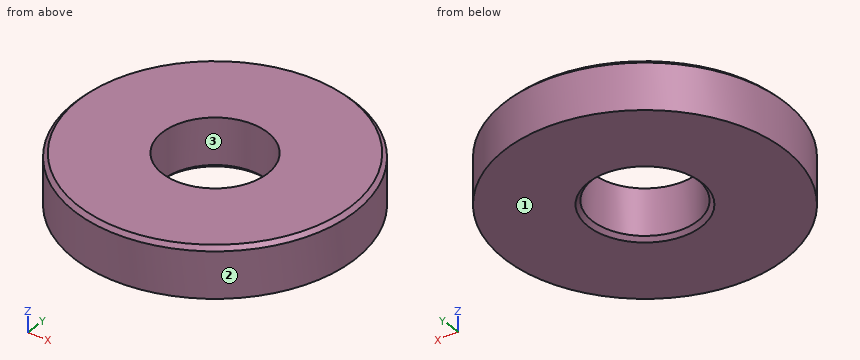
```python
from build123d import *

# Parameters (mm, degrees)
SKETCH_1_R      = 10.75
SKETCH_1_R_2    = 4.04
EXTRUDE_1_DEPTH = 3.85
CHAMFER_1_SIZE  = 0.3
CHAMFER_2_SIZE  = 0.3


with BuildPart() as part:
    # 草图1 → 凸台-拉伸1 (new body)
    with BuildSketch(Plane.XY):
        Circle(SKETCH_1_R)
        Circle(SKETCH_1_R_2, mode=Mode.SUBTRACT)
    extrude(amount=EXTRUDE_1_DEPTH)

    # 倒角1
    chamfer_1_edges = [part.edges().sort_by_distance(p)[0] for p in [
        (-10.75, 0, 3.85),
    ]]
    chamfer(chamfer_1_edges, length=CHAMFER_1_SIZE)

    # 倒角2
    chamfer_2_edges = [part.edges().sort_by_distance(p)[0] for p in [
        (-4.04, 0, 0),
    ]]
    chamfer(chamfer_2_edges, length=CHAMFER_2_SIZE)


solid = part.part
```
Source: CAD feature listing. Evaluate the final solid. Frame: model axes, mm. Face numbers are marked on the shaded views. Coordinates: 2 decimals unless noted, no trailing zeros. Loops run counter-clockwise (first coordinate to the right, second up) from the corner with the lowest first, then second, coordinate; pieces in that order, holes last. Notation, with made-up numbers: M 42.5,20 L 77.5,20 A15 ccw 77.5,34 Z; hole C 32.5,21.5 d2. An arc over 180 degrees is marked long. Put each result on its own line as item: value. Start each with the question number.
1) Cut plane C-C on z = 3.25. Return the cut outline in (x, y), then the cut area to 3 significant figures.
2) Ray query, L1, parallel to Y at x = 0, z = 3.05; L2, parallel to X at y = -0.25, z = 3.2; L3, parallel to X at y = 1, z = 3.5. Return the intervals inside material, ascending. Write a range as from..to.
3) Contact query for flat-ended pins moving along their axis: pin 1 Ø3 at (x, y) = (4, 3) entering from -Z; pin 2 Ø2 at (x, z) = (-3, 2) entering from +Y; pin 3 Ø1 at (x, z) = (2.5, 2) entering from -Y. Output: stop coordinate, or through.
4) Cut plane A-A on y = 0. Return the cut outline in (x, z), then the cut area to 3 significant figures.
5) Pull-direction query (X, two-part tool) for the marked faces 1, 2 and 3; classes: pulls with the +X half, pulls with the -X half, needs draft (parallel to the pull), parting line crosses it, or undercut.
The answers:
1. outline: C 0,0 d21.5; hole C 0,0 d8.08
1. area: 312 mm²
2. L1: y = -10.75..-4.04, 4.04..10.75
2. L2: x = -10.75..-4.03, 4.03..10.75
2. L3: x = -10.7..-3.91, 3.91..10.7
3. pin 1: stops at z = 0
3. pin 2: stops at y = 10.56
3. pin 3: stops at y = -10.56
4. outline: M -10.75,0 L -4.34,0 L -4.04,0.3 L -4.04,3.85 L -10.45,3.85 L -10.75,3.55 Z; M 4.04,0.3 L 4.34,0 L 10.75,0 L 10.75,3.55 L 10.45,3.85 L 4.04,3.85 Z
4. area: 51.5 mm²
5. face 1: needs draft
5. face 2: parting line crosses it
5. face 3: undercut
